CAD build for the part. Positions are in the model's coordinates, mm. Coordinates: 2 decimals unless noted, no trailing zeros. Write each loop counter-clockwise with the first axis right and the second up, starting at its lowest first coordinate (ties: lowest second). Pieces come first, ordered by that corner, then holes. Notation, with made-up numbers: (8.5, -34.75) - (58.5, -34.75) arc R20 cw to (58.5, -0.75) - close; hole circle Ø7 at (48, -35). An arc over 180 degrees is marked (long way). One line per question, with ' | ' between items. Start each with the question number.
1. Two-plate mould, pull along Z, no slides. Class faces 1 (the cylindrical face through (-6.572, 0.289, 24.508)), 2 (the cylindrical face through (-0.75, -5.7, 6.49)), 3 (the flat face through (2, -4, 30)): +Z half, -Z half, draft (parallel to the pull), parting line (faces both ways), or undercut.
2. Band-saw the part on A-A, the plane x = 0. Write the cut outline in (y, z).
3. Probe line 1 (Y direction, x = 0, z = 12); line 2 (X direction, y = -1.75, z = 28.5); line 3 (Y direction, x = 0, z = 7). List the from-to ranges inside material, lowest first.
4. Flat gauge pins, fed straight in: P1, Ø5, axis at y = -4.5, z = 3.5, coming from the -X side; P2, Ø1, axis at y = -3, z = 3.5, coming from the -X side; P3, Ø4, axis at x = 0.5, z = 22.5, coming from the +Y side. Where does each tip first touch, or does it go through?
5. Band-saw the part on C-C, the plane z = 13. Write the cut outline in (x, y), then the cut area to 3 significant figures.
from build123d import *

# Parameters (mm, degrees)
SKETCH_1_R          = 6.75
EXTRUDE_1_DEPTH     = 30
SKETCH_3_R          = 4
CUT_EXTRUDE_1_DEPTH = 32.482137793


# Read off the part's stored shape, not the designer's step: G1/4 直管螺纹 螺柱1
with BuildPart() as part:
    # 草图1 → 凸台-拉伸1 (new body)
    with BuildSketch(Plane.XY):
        Circle(SKETCH_1_R)
    extrude(amount=EXTRUDE_1_DEPTH)

    # 草图2 → 切除-旋转1 (revolve, cut)
    with BuildSketch(Plane(origin=(0, 0, 0), x_dir=(0, 0, -1), z_dir=(1, 0, 0)), mode=Mode.PRIVATE) as cut_revolve_1_sk:
        Polygon((-8, 6.75), (-7, 5.75), (-6, 5.75), (-5, 6.75), align=None)
    revolve(cut_revolve_1_sk.sketch.rotate(Axis((0, 0, 3.925992106), (0, 0, -1)), 90), axis=Axis((0, 0, 3.925992106), (0, 0, -1)), mode=Mode.SUBTRACT)

    # 草图3 → 切除-拉伸1 (cut, through all)
    with BuildSketch(Plane.XY.offset(30)):
        Circle(SKETCH_3_R)
    extrude(amount=-CUT_EXTRUDE_1_DEPTH, mode=Mode.SUBTRACT)

    # G1/4 直管螺纹 螺柱1 outline → G1/4 直管螺纹 螺柱1 (revolve, cut)
    with BuildSketch(Plane.XZ):
        Polygon((6.75, 30), (5.7225, 30), (6.5785, 29.144), (6.5785, 20), (6.75, 20), align=None)
    revolve(axis=Axis((0, 0, 0), (0, 0, 1)), mode=Mode.SUBTRACT)


solid = part.part
Filled in:
1) face 1: draft | face 2: undercut | face 3: +Z half
2) outline: (-6.75, 0) - (-4, 0) - (-4, 30) - (-5.72, 30) - (-6.58, 29.14) - (-6.58, 20) - (-6.75, 20) - (-6.75, 8) - (-5.75, 7) - (-5.75, 6) - (-6.75, 5) - close; (4, 0) - (6.75, 0) - (6.75, 5) - (5.75, 6) - (5.75, 7) - (6.75, 8) - (6.75, 20) - (6.58, 20) - (6.58, 29.14) - (5.72, 30) - (4, 30) - close
3) line 1: y = -6.75 to -4, 4 to 6.75 | line 2: x = -6.34 to -3.6, 3.6 to 6.34 | line 3: y = -5.75 to -4, 4 to 5.75
4) P1: stops at x = -6.45 | P2: stops at x = -6.27 | P3: stops at y = 6.58
5) outline: circle Ø13.5 at (0, 0); hole circle Ø8 at (0, 0) | area: 92.9 mm²
